```python
from build123d import *

# Parameters (mm, degrees)
SKETCH1_W           = 50.8
SKETCH1_H           = 50.8
BOSS_EXTRUDE1_DEPTH = 1.5875
FILLET1_R           = 2.54
SKETCH2_R           = 2.032
CUT_EXTRUDE1_DEPTH  = 37.061067996


with BuildPart() as part:
    # Sketch1 → Boss-Extrude1 (new, symmetric)
    with BuildSketch(Plane.XY):
        Rectangle(SKETCH1_W, SKETCH1_H)
    extrude(amount=BOSS_EXTRUDE1_DEPTH, both=True)

    # Fillet1
    fillet1_edges = [part.edges().sort_by_distance(p)[0] for p in [
        (25.4, -25.4, 0),
        (-25.4, -25.4, 0),
        (-25.4, 25.4, 0),
        (25.4, 25.4, 0),
    ]]
    fillet(fillet1_edges, radius=FILLET1_R)

    # Sketch2 → Cut-Extrude1 (cut, through all)
    with BuildSketch(Plane.XY.offset(1.5875)):
        with Locations((-12.7, 12.7)):
            Circle(SKETCH2_R)
        with Locations((0, 12.7)):
            Circle(SKETCH2_R)
        with Locations((12.7, 12.7)):
            Circle(SKETCH2_R)
        with Locations(Location((12.7, -12.7, 0), (0, 0, 180))):
            Circle(SKETCH2_R)
        with Locations(Location((0, -12.7, 0), (0, 0, 180))):
            Circle(SKETCH2_R)
        with Locations(Location((-12.7, -12.7, 0), (0, 0, 180))):
            Circle(SKETCH2_R)
    extrude(amount=-CUT_EXTRUDE1_DEPTH, mode=Mode.SUBTRACT)


solid = part.part
```
For this review, take the finished solid that the model builds, in its own axes (mm). Round coordinates to 2 decimals unless told otherwise and drop trailing zeros. Write each loop counter-clockwise with the first axis right and the second up, starting at its lowest first coordinate (ties: lowest second). Pieces come first, ordered by that corner, then holes.
1) Mouldability with a two-part tool opening along Y and no side actions: class faces 1 (the face through (-24.676, -24.636, 0.022)), 2 (the face through (0, 0, 1.588)), 3 (the face through (-0.44, 10.716, 0.022)) as +Y half, -Y half, draft (parallel to the pull), parting line (faces both ways), or undercut.
Answer below:
face 1: -Y half
face 2: draft
face 3: undercut
2) Take a section at A-A on z = -0.9. Give the boundary of the cut face in (x, y), then the cut area to 3 significant figures.
Answer below:
outline: (-25.4, -22.86) arc R2.54 ccw to (-22.86, -25.4) - (22.86, -25.4) arc R2.54 ccw to (25.4, -22.86) - (25.4, 22.86) arc R2.54 ccw to (22.86, 25.4) - (-22.86, 25.4) arc R2.54 ccw to (-25.4, 22.86) - close; hole circle Ø4.06 at (-12.7, -12.7); hole circle Ø4.06 at (-12.7, 12.7); hole circle Ø4.06 at (0, -12.7); hole circle Ø4.06 at (0, 12.7); hole circle Ø4.06 at (12.7, -12.7); hole circle Ø4.06 at (12.7, 12.7)
area: 2,500 mm2
3) Insertion check: pin 1 Ø2.5 at (x, y) = (12.7, 12.7) entering from -Z. The pin has a flat end and moves straight along its axis. Give the tip position at first contact, or say it passes through.
Answer below:
pin 1: passes through
4) For line 1 along Y through (x, z) = (0, -0.4); line 2 along X through (y, z) = (-12.7, -0.2); line 3 along Y through (x, z) = (14, -0.9), list the stretches that pass through material, from the lowest coordinate up.
Answer below:
line 1: y = -25.4 to -14.73, -10.67 to 10.67, 14.73 to 25.4
line 2: x = -25.4 to -14.73, -10.67 to -2.03, 2.03 to 10.67, 14.73 to 25.4
line 3: y = -25.4 to -14.26, -11.14 to 11.14, 14.26 to 25.4
5) Take a section at B-B on y = -12.7. Give the boundary of the cut face in (x, z), then the cut area to 3 significant figures.
Answer below:
outline: (-25.4, -1.59) - (-14.73, -1.59) - (-14.73, 1.59) - (-25.4, 1.59) - close; (-10.67, -1.59) - (-2.03, -1.59) - (-2.03, 1.59) - (-10.67, 1.59) - close; (2.03, -1.59) - (10.67, -1.59) - (10.67, 1.59) - (2.03, 1.59) - close; (14.73, -1.59) - (25.4, -1.59) - (25.4, 1.59) - (14.73, 1.59) - close
area: 123 mm2
6) Take a section at C-C on x = 0. Give the boundary of the cut face in (y, z).
Answer below:
outline: (-25.4, -1.59) - (-14.73, -1.59) - (-14.73, 1.59) - (-25.4, 1.59) - close; (-10.67, -1.59) - (10.67, -1.59) - (10.67, 1.59) - (-10.67, 1.59) - close; (14.73, -1.59) - (25.4, -1.59) - (25.4, 1.59) - (14.73, 1.59) - close
